```python
from build123d import *

# Parameters (mm, degrees)
SKETCH1_R           = 1.5
BOSS_EXTRUDE1_DEPTH = 1.35
CHAMFER1_SIZE       = 0.4


with BuildPart() as part:
    # Sketch1 → Boss-Extrude1 (new body, symmetric)
    with BuildSketch(Plane(origin=(0, 0, 0), x_dir=(1, 0, 0), z_dir=(0, 1, 0))):
        with BuildLine():
            Line((-13.25, 3.25), (13.25, 3.25))
            ThreePointArc((13.25, 3.25), (16.5, 0), (13.25, -3.25))
            Line((13.25, -3.25), (-13.25, -3.25))
            ThreePointArc((-13.25, -3.25), (-16.5, 0), (-13.25, 3.25))
        make_face()
        with Locations((-13.25, 0)):
            Circle(SKETCH1_R, mode=Mode.SUBTRACT)
        with Locations((13.25, 0)):
            Circle(SKETCH1_R, mode=Mode.SUBTRACT)
    extrude(amount=BOSS_EXTRUDE1_DEPTH, both=True)

    # Chamfer1
    chamfer1_edges = [part.edges().sort_by_distance(p)[0] for p in [
        (16.5, 1.35, 0),
        (0, 1.35, -3.25),
        (-16.5, 1.35, 0),
        (0, 1.35, 3.25),
    ]]
    chamfer(chamfer1_edges, length=CHAMFER1_SIZE)


solid = part.part
```
The model under review builds one solid part; all positions refer to its coordinate system, in mm. Round coordinates to 2 decimals unless told otherwise and drop trailing zeros. Order: outer loops, then holes, each group sorted by start corner. A loop starts at its lowest first (then second) coordinate and runs counter-clockwise, first axis right, second up. Notation, with made-up numbers: (-4, -14) - (50, -14) arc R22 cw to (50, 18) - close; hole circle Ø7 at (41, 10.25). An arc over 180 degrees is marked (long way). Answer in a Markdown table with one row per item.
(1) Mouldability with a two-part tool opening along X and no side actions: class faces 1 (the face through (-14.75, -0.02, -0.07)), 2 (the face through (0, 0, -3.25)), 3 (the face through (16.5, -0.2, -0.1)) as released by +X, released by -X, zero draft, split by the parting line, or undercut.
Result set:
| item | result |
|---|---|
| face 1 | undercut |
| face 2 | zero draft |
| face 3 | released by +X |
(2) For line 1 (X direction, y = 0.05, z = 0); line 2 (X direction, y = 0.8, z = -0.75); line 3 (Z direction, x = 13.25, y = -0.1), list the stretches that pass through material, from the lowest coordinate up. Write a range as from..to.
Result set:
| item | result |
|---|---|
| line 1 | x = -16.5..-14.75, -11.75..11.75, 14.75..16.5 |
| line 2 | x = -16.41..-14.55, -11.95..11.95, 14.55..16.41 |
| line 3 | z = -3.25..-1.5, 1.5..3.25 |
(3) Clearance check with flat-ended pins moving along their axes: P1, Ø3.5, axis at x = 13.25, z = 0, coming from the +Y side; P2, Ø1, axis at y = 1, z = 2, coming from the +X side. State where each tip first meets the part, or that it passes through.
Result set:
| item | result |
|---|---|
| P1 | stops at y = 1.35 |
| P2 | stops at x = 16.13 |
(4) Take a section at A-A on x = 12.5. Write out the cut boundary in (y, z), plus the area to 3 significant figures.
Result set:
| item | result |
|---|---|
| outline | (-1.35, -3.25) - (0.95, -3.25) - (1.35, -2.85) - (1.35, -1.3) - (-1.35, -1.3) - close; (-1.35, 1.3) - (1.35, 1.3) - (1.35, 2.85) - (0.95, 3.25) - (-1.35, 3.25) - close |
| area | 10.4 mm2 |
(5) Take a section at C-C on z = 1. Count the separate pieces of the cut face and the enclosed holes in it, plus the area to 3 significant figures.
Result set:
| item | result |
|---|---|
| separate pieces | 3 |
| enclosed holes | 0 |
| area | 76.0 mm2 |
(6) Take a section at B-B on y = -0.7. Write out the cut boundary in (x, z).
Result set:
| item | result |
|---|---|
| outline | (-13.25, -3.25) - (13.25, -3.25) arc R3.25 ccw to (13.25, 3.25) - (-13.25, 3.25) arc R3.25 ccw to start; hole circle Ø3 at (-13.25, 0); hole circle Ø3 at (13.25, 0) |
